The listing builds one solid part. Answer for the finished solid, in the listing's coordinates (mm). Coordinates: 2 decimals unless noted, no trailing zeros. Loops run counter-clockwise (first coordinate to the right, second up) from the corner with the lowest first, then second, coordinate; pieces in that order, holes last. Notation, with made-up numbers: (24.25, 19.25) - (71.25, 19.25) arc R27 ccw to (71.25, 54.25) - close; hole circle Ø3 at (89.25, -32.75). An arc over 180 degrees is marked (long way). Return JSON: item names as keys, results as strings. Group by question number.
1. Find the intervals of material crossed by line 1 along Y through (x, z) = (-15, 0.3); line 2 along X through (y, z) = (5, 2.35); line 3 along X through (y, z) = (13, 2.95), in increasing order.
2. Each of these flat-tipped pins is pushed along its axis until it touches: P1, Ø1.5, axis at x = 15.5, z = 2, coming from the +Y side; P2, Ø1.5, axis at y = 10, z = 1, coming from the +X side; P3, Ø12, axis at x = 7.5, y = -11, coming from the +Z side. Where does it stop, or does it pass through?
3. The mould has two halves that part along X. Classify faces 1 (the face through (20.03, 6.31, 3.26)), 2 (the face through (-20.633, -15.821, 0.991)), 3 (the face through (-6, 21, 0)): pulls with the +X half, pulls with the -X half, needs draft (parallel to the pull), parting line crosses it, or undercut.
4. Section A-A (y = 0) is taken. Write down the section's boundary in (x, z), and give its area (3 significant figures).
5. Section C-C (z = 2.95) is taken. Write down the section's boundary in (x, y).
```python
from build123d import *

# Parameters (mm, degrees)
SKETCH052_R     = 26
SKETCH052_R_2   = 21
PAD034_DEPTH    = 6
CHAMFER016_SIZE = 3.99
CHAMFER017_SIZE = 0.6


with BuildPart() as part:
    # Sketch052 (on XY_Plane016 of Origin031) → Pad034 (new body)
    with BuildSketch(Plane.XY):
        Circle(SKETCH052_R)
        Circle(SKETCH052_R_2, mode=Mode.SUBTRACT)
    extrude(amount=PAD034_DEPTH)

    # Chamfer016
    chamfer016_edges = [part.edges().sort_by_distance(p)[0] for p in [
        (-26, 0, 6),
    ]]
    chamfer(chamfer016_edges, length=CHAMFER016_SIZE)

    # Chamfer017
    chamfer017_edges = [part.edges().sort_by_distance(p)[0] for p in [
        (-21, 0, 0),
    ]]
    chamfer(chamfer017_edges, length=CHAMFER017_SIZE)


solid = part.part
```
The answers:
{
 "1": {"line 1": "y = -21.24 to -15.12, 15.12 to 21.24", "line 2": "x = -25.17 to -20.4, 20.4 to 25.17", "line 3": "x = -21.42 to -16.49, 16.49 to 21.42"},
 "2": {"P1": "stops at y = 21.41", "P2": "stops at x = 24.3", "P3": "passes through"},
 "3": {"face 1": "undercut", "face 2": "parting line crosses it", "face 3": "needs draft"},
 "4": {"outline": "(-26, 0) - (-21.6, 0) - (-21, 0.6) - (-21, 6) - (-22.01, 6) - (-26, 2.01) - close; (21, 0.6) - (21.6, 0) - (26, 0) - (26, 2.01) - (22.01, 6) - (21, 6) - close", "area": "43.7 mm2"},
 "5": {"outline": "circle Ø50.12 at (0, 0); hole circle Ø42 at (0, 0)"}
}
